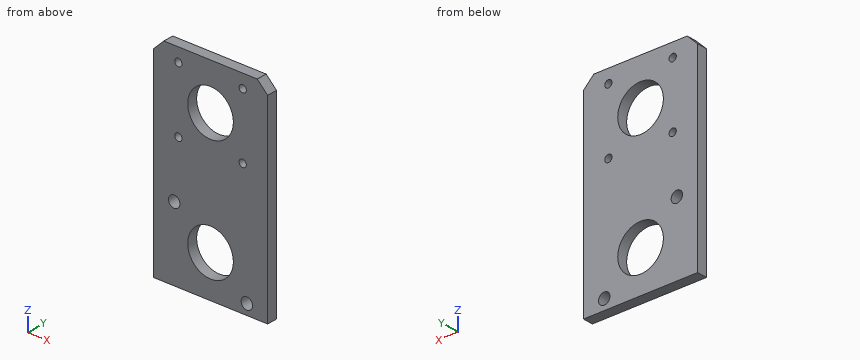
```python
from build123d import *

# Parameters (mm, degrees)
F0_W     = 55
F0_H     = 100
F0_R     = 2.75
F0_R_2   = 11
F0_R_3   = 1.75
F1_DEPTH = 5
F2_SIZE  = 5
F3_SIZE  = 5


with BuildPart() as f1:
    # F0 (on Front) → F1 (new body)
    with BuildSketch(Plane.XZ):
        Rectangle(F0_W, F0_H)
        with Locations((-17.5, -15)):
            Circle(F0_R, mode=Mode.SUBTRACT)
        with Locations((0, -30)):
            Circle(F0_R_2, mode=Mode.SUBTRACT)
        with Locations((17.5, -45)):
            Circle(F0_R, mode=Mode.SUBTRACT)
        with Locations((-15.5, 12.5)):
            Circle(F0_R_3, mode=Mode.SUBTRACT)
        with Locations((-15.5, 43.5)):
            Circle(F0_R_3, mode=Mode.SUBTRACT)
        with Locations((15.5, 12.5)):
            Circle(F0_R_3, mode=Mode.SUBTRACT)
        with Locations((0, 28)):
            Circle(F0_R_2, mode=Mode.SUBTRACT)
        with Locations((15.5, 43.5)):
            Circle(F0_R_3, mode=Mode.SUBTRACT)
    extrude(amount=F1_DEPTH)

    # F2
    f2_edges = [f1.edges().sort_by_distance(p)[0] for p in [
        (-27.5, -2.5, 50),
    ]]
    chamfer(f2_edges, length=F2_SIZE)

    # F3
    f3_edges = [f1.edges().sort_by_distance(p)[0] for p in [
        (27.5, -2.5, 50),
    ]]
    chamfer(f3_edges, length=F3_SIZE)


solid = f1.part
```
Design review of the part built by this model. Coordinates are the model's own, in mm. Coordinates: 2 decimals unless noted, no trailing zeros. Loops run counter-clockwise (first coordinate to the right, second up) from the corner with the lowest first, then second, coordinate; pieces in that order, holes last. Notation, with made-up numbers: M 88.25,-10 L 128.25,-10 A13 ccw 128.25,6 Z; hole C 11.5,81 d5. An arc over 180 degrees is marked long. One line per question, with ' | ' between items.
(1) Wall thickness on probe 1 along Z at (x, y) = (-1, -2); probe 2 along Z at (x, y) = (3, -1.7); probe 3 along Z at (x, y) = (15.5, -3.9): over which ranges is each line inside the solid? List them lowest first.
Filled in:
probe 1: z = -50 to -40.95, -19.05 to 17.05, 38.95 to 50 | probe 2: z = -50 to -40.58, -19.42 to 17.42, 38.58 to 50 | probe 3: z = -50 to -46.89, -43.11 to 10.75, 14.25 to 41.75, 45.25 to 50
(2) We need section C-C (z = -45). Give the boundary of the cut face in (x, y), and give its area (4 significant figures).
Filled in:
outline: M -27.5,-5 L 14.75,-5 L 14.75,0 L -27.5,0 Z; M 20.25,-5 L 27.5,-5 L 27.5,0 L 20.25,0 Z | area: 247.5 mm^2
(3) We need section A-A (z = 12.5). Give the boundary of the cut face in (x, y).
Filled in:
outline: M -27.5,-5 L -17.25,-5 L -17.25,0 L -27.5,0 Z; M -13.75,-5 L 13.75,-5 L 13.75,0 L -13.75,0 Z; M 17.25,-5 L 27.5,-5 L 27.5,0 L 17.25,0 Z
(4) We need section D-D (y = -3.75). Count the separate pieces of the cut face and the enclosed holes in it, and give its area (3 significant figures).
Filled in:
separate pieces: 1 | enclosed holes: 8 | area: 4,630 mm^2
(5) We need section B-B (x = -5). Give the boundary of the cut face in (y, z), and give its area (3 significant figures).
Filled in:
outline: M -5,-50 L 0,-50 L 0,-39.8 L -5,-39.8 Z; M -5,-20.2 L 0,-20.2 L 0,18.2 L -5,18.2 Z; M -5,37.8 L 0,37.8 L 0,50 L -5,50 Z | area: 304 mm^2
